from build123d import *

# Parameters (mm, degrees)
F1_DEPTH = 25
F3_DEPTH = 25


with BuildPart() as f1:
    # F0 (on Front) → F1 (new body)
    with BuildSketch(Plane.XZ):
        with BuildLine():
            Line((2.366019, 5.866973), (-47.633981, 5.866973))
            Line((-47.633981, 5.866973), (-47.633981, -4.133027))
            Line((-47.633981, -4.133027), (2.366019, -4.133027))
            ThreePointArc((2.366019, -4.133027), (7.366019, 0.866973), (2.366019, 5.866973))
        make_face()
        with BuildLine():
            ThreePointArc((2.366019, 3.449053), (4.948099, 0.866973), (2.366019, -1.715107))
            Line((2.366019, -1.715107), (-17.543796, -1.715107))
            ThreePointArc((-17.543796, -1.715107), (-20.125876, 0.866973), (-17.543796, 3.449053))
            Line((-17.543796, 3.449053), (2.366019, 3.449053))
        make_face(mode=Mode.SUBTRACT)
    extrude(amount=F1_DEPTH)

    # F2 (on face) → F3 (join)
    with BuildSketch(Plane.XZ.offset(25)):
        Polygon((-28.071029, 1.708739), (-47.633981, 5.866973), (-47.633981, -4.133027), (-28.071029, 0.025206), align=None)
    extrude(amount=F3_DEPTH)


solid = f1.part
Check sheet for the modelled part. Datum: model origin and axes. Units: mm. A direction names the side the tool comes from. Round coordinates to 2 decimals unless told otherwise and drop trailing zeros. Order: outer loops, then holes, each group sorted by start corner. A loop starts at its lowest first (then second) coordinate and runs counter-clockwise, first axis right, second up.
(1) Draft check along X on faces 4 (the cylindrical face through (7.365, -12.325, 0.757)), 5 (the cylindrical face through (-20.125, -12.325, 0.81)), 6 (the flat face through (-47.634, -25, 1)), 7 (the flat face through (-27, 0, 1)). Enter one of: pulls with the +X half, pulls with the -X half, needs draft (parallel to the pull), parting line crosses it, or undercut.
(2) Access from +Z, -Z, +X, -X, +Y, -Y to the whole of each face (thin tool, end or side, straight path). Record for faces 1 (the cylindrical face through (4.947, -12.325, 0.924)), 2 (the flat face through (-37.989, -37.325, -2.083)), 3 (the flat face through (-28.071, -37, 1)).
(3) Cross-section at D-D, the plane x = -19. Enter the section's corners in (y, z).
(4) Cross-section at A-A, the plane x = -9.5. Enter the section's corners in (y, z).
(5) Cross-section at C-C, the plane z = 0.75. Enter the section's corners in (x, y).
(6) Go/stop test with flat-tipped pins: P1, Ø0.5, axis at y = -38, z = 1, coming from the +X side; P2, Ø8, axis at x = -23.5, y = -41.5, coming from the -Z side. Record where each tip stops, or that it passes through.
(7) Scan lines: probe 1 along Z at (x, y) = (-11.5, -17.5); probe 2 along Y at (x, z) = (-25.5, 2.5); probe 3 along X at (y, z) = (-12, -0.75). Record each from-to range of solid material in increasing order.
(8) Cross-section at B-B, the plane y = -5. Enter the section's corners in (x, z), and give its area (3 significant figures).
Check sheet entries:
1. face 4: pulls with the +X half
1. face 5: undercut
1. face 6: pulls with the -X half
1. face 7: needs draft
2. face 1: +Y, -Y
2. face 2: -Z, +X, -Y
2. face 3: +Z, -Z, +X, -Y
3. outline: (-25, -4.13) - (0, -4.13) - (0, -1.27) - (-25, -1.27) - close; (-25, 3) - (0, 3) - (0, 5.87) - (-25, 5.87) - close
4. outline: (-25, -4.13) - (0, -4.13) - (0, -1.72) - (-25, -1.72) - close; (-25, 3.45) - (0, 3.45) - (0, 5.87) - (-25, 5.87) - close
5. outline: (-47.63, -50) - (-28.07, -50) - (-28.07, -25) - (-20.12, -25) - (-20.12, 0) - (-47.63, 0) - close; (4.95, -25) - (7.36, -25) - (7.36, 0) - (4.95, 0) - close
6. P1: stops at x = -28.07
6. P2: passes through
7. probe 1: z = -4.13 to -1.72, 3.45 to 5.87
7. probe 2: y = -25 to 0
7. probe 3: x = -47.63 to -19.56, 4.38 to 7.1
8. outline: (-47.63, -4.13) - (2.37, -4.13) arc R5 ccw to (2.37, 5.87) - (-47.63, 5.87) - close; hole (-17.54, -1.72) - (2.37, -1.72) arc R2.58 ccw to (2.37, 3.45) - (-17.54, 3.45) arc R2.58 ccw to start
8. area: 416 mm2
